The model under review builds one solid part; all positions refer to its coordinate system, in mm. A direction names the side the tool comes from. Round coordinates to 2 decimals unless told otherwise and drop trailing zeros. Order: outer loops, then holes, each group sorted by start corner. A loop starts at its lowest first (then second) coordinate and runs counter-clockwise, first axis right, second up. Notation, with made-up numbers: M 38,73.5 L 87,73.5 A27 cw 87,108.5 Z; hole C 15.5,86 d5. An arc over 180 degrees is marked long. Answer as a JSON object with one key per item and string values. Group by question number.
1. Add section B-B on x = 31.75. State the section outline as (y, z) points (1 decimal), and give its area (3 significant figures).
2. Clearance check with flat-ended pins moving along their axes: P1, Ø0.5, axis at y = 20.5, z = 9, coming from the +X side; P2, Ø3.5, axis at x = -0.5, z = 7, coming from the +Y side; P3, Ø0.8, axis at y = 20, z = 7, coming from the -X side. State where each tip first meets the part, or that it passes through.
3. To check wall thickness, follow probe 1 along X at (y, z) = (31.75, 10.3); probe 2 along X at (y, z) = (35.5, 9.75); probe 3 along Y at (x, z) = (-9, 9.75). State the ranges of each line that lie inside material, in increasing order. Write a range as [from, to].
4. Add section D-D on y = 35.75. State the section outline as (x, z) points (3 decimals), and give its area (3 significant figures).
5. Mouldability with a two-part tool opening along Y and no side actions: class faces 4 (the face through (37.26, 33.49, 11.09)), 5 (the face through (2.05, 20, 9)), 6 (the face through (0, 22.606, 10)), 7 (the face through (-5.27, 20.41, 7.18)) as released by +Y, released by -Y, zero draft, split by the parting line, or undercut.
6. Add section A-A on y = 31.75. State the section outline as (x, z) points (1 decimal), and give its area (3 significant figures).
7. Machinability: for faces 1 (the face through (26, 26, 9.525)), 2 (the face through (-26, 27, 9.525)), 3 (the face through (-23.133, 24.61, 11.09)), which of the approach directions +Z, -Z, +X, -X, +Y, -Y give a long, thin tool a straight path to every point of the face, cutting with its end or side? Answer none if there is none.
8. Add section C-C on z = 10.75. State the section outline as (x, y) points, and give its area (3 significant figures).
```python
from build123d import *

# Parameters (mm, degrees)
SKETCH1_R                      = 5.7785
SKETCH1_W                      = 4.1
SKETCH1_H                      = 1.651
BOSS_EXTRUDE1_DEPTH            = 12.7
CUT_EXTRUDE1_REACH             = 6.445
CUT_EXTRUDE1_DIRECTION_2_DEPTH = 18.4625


with BuildPart() as part:
    # Sketch1 → Boss-Extrude1 (new body)
    with BuildSketch(Plane.XY):
        with BuildLine():
            Line((-22.056518803, 18.161), (22.056518803, 18.161))
            ThreePointArc((22.056518803, 18.161), (31.546886224, 20.574211288), (38.731794688, 27.227612888))
            ThreePointArc((38.731794688, 27.227612888), (32.803412582, 40.00153102), (23.855967837, 29.126700844))
            ThreePointArc((23.855967837, 29.126700844), (23.171856155, 24.662896524), (19.151565806, 22.606))
            Line((19.151565806, 22.606), (-19.151565806, 22.606))
            ThreePointArc((-19.151565806, 22.606), (-23.171856155, 24.662896524), (-23.855967837, 29.126700844))
            ThreePointArc((-23.855967837, 29.126700844), (-32.803412582, 40.00153102), (-38.731794688, 27.227612888))
            ThreePointArc((-38.731794688, 27.227612888), (-31.546886224, 20.574211288), (-22.056518803, 18.161))
        make_face()
        with Locations((-31.75, 31.75)):
            Circle(SKETCH1_R, mode=Mode.SUBTRACT)
        with Locations((31.75, 31.75)):
            Circle(SKETCH1_R, mode=Mode.SUBTRACT)
        with Locations((0, 20.2565)):
            Rectangle(SKETCH1_W, SKETCH1_H, mode=Mode.SUBTRACT)
    extrude(amount=BOSS_EXTRUDE1_DEPTH)

    # Sketch2 → Cut-Extrude1 (cut, up to next)
    with BuildSketch(Plane(origin=(0, 22.606, 0), x_dir=(1, 0, 0), z_dir=(0, 1, 0)), mode=Mode.PRIVATE) as cut_extrude1_sk1:
        Polygon((-46.157400287, -9.525), (-6.524655543, -9.525), (-3.978583924, -4.7625), (3.978583924, -4.7625), (6.524655543, -9.525), (46.157400287, -9.525), (46.157400287, 7.651360298), (-46.157400287, 7.651360298), align=None)
    cut_extrude1_tool1 = extrude(cut_extrude1_sk1.sketch, amount=-CUT_EXTRUDE1_REACH, mode=Mode.PRIVATE) & part.part
    add(cut_extrude1_tool1.solids().sort_by_distance((0, 22.606, 0.728365))[0], mode=Mode.SUBTRACT)

    # Sketch2 → Cut-Extrude1 direction 2 (cut)
    with BuildSketch(Plane(origin=(0, 22.606, 0), x_dir=(1, 0, 0), z_dir=(0, 1, 0))):
        Polygon((-46.157400287, -9.525), (-6.524655543, -9.525), (-3.978583924, -4.7625), (3.978583924, -4.7625), (6.524655543, -9.525), (46.157400287, -9.525), (46.157400287, 7.651360298), (-46.157400287, 7.651360298), align=None)
    extrude(amount=CUT_EXTRUDE1_DIRECTION_2_DEPTH, mode=Mode.SUBTRACT)


solid = part.part
```
Recorded:
{
 "1": {"outline": "M 20.7,9.5 L 26,9.5 L 26,12.7 L 20.7,12.7 Z; M 37.5,9.5 L 40.1,9.5 L 40.1,12.7 L 37.5,12.7 Z", "area": "24.8 mm²"},
 "2": {"P1": "stops at x = 6.38", "P2": "stops at y = 22.61", "P3": "stops at x = -5.39"},
 "3": {"probe 1": "x = [-40.07, -37.53], [-25.97, -23.43], [23.43, 25.97], [37.53, 40.07]", "probe 2": "x = [-39.18, -36.15], [-27.35, -24.32], [24.32, 27.35], [36.15, 39.18]", "probe 3": "y = [18.16, 22.61]"},
 "4": {"outline": "M -39.044,9.525 L -35.92,9.525 L -35.92,12.7 L -39.044,12.7 Z; M -27.58,9.525 L -24.456,9.525 L -24.456,12.7 L -27.58,12.7 Z; M 24.456,9.525 L 27.58,9.525 L 27.58,12.7 L 24.456,12.7 Z; M 35.92,9.525 L 39.044,9.525 L 39.044,12.7 L 35.92,12.7 Z", "area": "39.7 mm²"},
 "5": {"face 4": "undercut", "face 5": "undercut", "face 6": "released by +Y", "face 7": "zero draft"},
 "6": {"outline": "M -40.1,9.5 L -37.5,9.5 L -37.5,12.7 L -40.1,12.7 Z; M -26,9.5 L -23.4,9.5 L -23.4,12.7 L -26,12.7 Z; M 23.4,9.5 L 26,9.5 L 26,12.7 L 23.4,12.7 Z; M 37.5,9.5 L 40.1,9.5 L 40.1,12.7 L 37.5,12.7 Z", "area": "32.3 mm²"},
 "7": {"face 1": "-Z, +X, +Y, -Y", "face 2": "-Z, -X, +Y, -Y", "face 3": "+Z, -Z"},
 "8": {"outline": "M -38.73,27.23 A19.87 ccw -22.06,18.16 L 22.06,18.16 A19.87 ccw 38.73,27.23 A8.32 ccw long 23.86,29.13 A4.96 cw 19.15,22.61 L -19.15,22.61 A4.96 cw -23.86,29.13 A8.32 ccw long Z; hole C -31.75,31.75 d11.56; hole M -2.05,19.43 L 2.05,19.43 L 2.05,21.08 L -2.05,21.08 Z; hole C 31.75,31.75 d11.56", "area": "545 mm²"}
}
